Autodesk Fusion 360 part; units mm, degrees
sketch "Sketch1" plane through (0, 0, 0) normal (0, 0, 1) x (1, 0, 0)
  line L0 (-35.5, 0) -> (-21.5, 0)
  line L1 (-21.5, 0) -> (-21.5, 44)
  line L2 (-21.5, 44) -> (21.5, 44)
  line L3 (21.5, 44) -> (21.5, 0)
  line L4 (21.5, 0) -> (35.5, 0)
  line L5 (35.5, 0) -> (35.5, 4)
  line L6 (35.5, 4) -> (25.5, 4)
  line L7 (25.5, 4) -> (25.5, 47)
  line L8 (25.5, 47) -> (-25.5, 47)
  line L9 (-25.5, 47) -> (-25.5, 4)
  line L10 (-25.5, 4) -> (-35.5, 4)
  line L11 (-35.5, 4) -> (-35.5, 0)
  dimension "d1" = 43
  dimension "d2" = 21.5
  dimension "d3" = 4
  dimension "d4" = 4
  dimension "d5" = 3
  dimension "d6" = 4
  dimension "d7" = 4
  dimension "d8" = 10
  dimension "d9" = 10
  dimension "d42" = 44
  dimension "d43" = 44
extrude "Extrude1" add sketch "Sketch1" along normal blind 43
sketch "Sketch3" plane through (0, 44, 0) normal (0, -1, 0) x (1, 0, 0)
  line L0 (-21.5, 0) -> (21.5, 0)
  line L1 (21.5, 0) -> (21.5, 43)
  line L2 (21.5, 43) -> (-21.5, 43)
  line L3 (-21.5, 43) -> (-21.5, 0)
  circle A0 centre (-15.5, 6) radius 1.65
  circle A1 centre (15.5, 6) radius 1.65
  circle A2 centre (-15.5, 37) radius 1.65
  circle A3 centre (15.5, 37) radius 1.65
  dimension "d14" = 3.3
  dimension "d15" = 6
  dimension "d16" = 6
  dimension "d19" = 31
  dimension "d20" = 31
extrude "Extrude2" cut sketch "Sketch3" against normal up to surface (3 mm away) contours A0 | A1 | A2 | A3
chamfer "Chamfer1" distance 5 angle 45 2 edges at (25.5, 4, 21.5) (-25.5, 4, 21.5)
sketch "Sketch5" plane through (0, 44, 0) normal (0, -1, 0) x (1, 0, 0)
  circle A0 centre (15.5, 37) radius 1.65
  circle A1 centre (15.5, 6) radius 1.65
  circle A2 centre (-15.5, 37) radius 1.65
  circle A3 centre (-15.5, 6) radius 1.65
  line L0 (-21.5, 0) -> (21.5, 0)
  line L1 (21.5, 0) -> (21.5, 43)
  line L2 (21.5, 43) -> (-21.5, 43)
  line L3 (-21.5, 43) -> (-21.5, 0)
  circle A4 centre (0, 21) radius 13
  dimension "d25" = 26
  dimension "d26" = 21.5
extrude "Extrude3" cut sketch "Sketch5" against normal up to surface (3 mm away) contours A4
sketch "Sketch6" plane through (0, 0, 0) normal (0, -1, 0) x (1, 0, 0)
  line L0 (21.5, 0) -> (35.5, 0)
  line L1 (35.5, 0) -> (35.5, 43)
  line L2 (35.5, 43) -> (21.5, 43)
  line L3 (21.5, 43) -> (21.5, 0)
  circle A0 centre (31.5, 36.6) radius 1.65
  circle A1 centre (-31.5, 36.6) radius 1.65
  line L4 (-21.5, 0) -> (-21.5, 43)
  line L5 (-35.5, 43) -> (-21.5, 43)
  circle A2 centre (31.5, 6.6) radius 1.65
  circle A3 centre (-31.5, 6.6) radius 1.65
  dimension "d29" = 3.3
  dimension "d30" = 10
  dimension "d31" = 3.3
  dimension "d32" = 10
  dimension "d33" = 6.4
  dimension "d34" = 6.4
  dimension "d37" = 0
  dimension "d38" = -30
extrude "Extrude4" cut sketch "Sketch6" against normal blind 10 contours A0 | A1 | A2 | A3
sketch "Sketch7" plane through (0, 4, 0) normal (0, 1, 0) x (-1, 0, 0)
  arc A0 (-30.5, 7.9124) -> (-30.5, 5.2876) centre (-31.5, 6.6) ccw
  line L0 (-30.5, 7.9124) -> (-30.5, 35.2876)
  arc A1 (-30.5, 37.9124) -> (-30.5, 35.2876) centre (-31.5, 36.6) ccw
  line L1 (-30.5, 37.9124) -> (-30.5, 43)
  line L2 (-30.5, 43) -> (-35.5, 43)
  line L3 (-35.5, 43) -> (-35.5, 0)
  line L4 (-35.5, 0) -> (-30.5, 0)
  line L5 (-30.5, 0) -> (-30.5, 5.2876)
  circle A2 centre (-31.5, 6.6) radius 4
  circle A3 centre (31.5, 6.6) radius 4
  circle A4 centre (-31.5, 36.6) radius 4
  circle A5 centre (31.5, 36.6) radius 4
  dimension "d44" = 8
  dimension "d47" = 63
  dimension "d48" = 30
extrude "Extrude5" cut sketch "Sketch7" along normal blind 4 contours A0 L0 L5 A2 | A0 L0 L5 A2 | L0 A1 L1 A4 | L0 A1 L1 A4 | A3 | A5
sketch "Sketch8" plane through (25.5, 0, 0) normal (1, 0, 0) x (0, 0, -1)
  line L0 (-43, 9) -> (0, 9)
  line L1 (0, 9) -> (0, 47)
  line L2 (0, 47) -> (-43, 47)
  line L3 (-43, 47) -> (-43, 9)
  line L4 (-26.5, 37) -> (-26.5, 19)
  arc A0 (-26.5, 19) -> (-16.5, 19) centre (-21.5, 19) ccw
  line L5 (-16.5, 19) -> (-16.5, 37)
  arc A1 (-16.5, 37) -> (-26.5, 37) centre (-21.5, 37) ccw
  line L6 (-21.5, 37) -> (-21.5, 19) construction
  dimension "d51" = 18
  dimension "d52" = 10
  dimension "d53" = 21.5
extrude "Extrude6" cut sketch "Sketch8" against normal up to surface (51 mm away) contours L4 A0 L5 A1
equation "d1 = size"
equation "d2 = d1 / 2"
equation "d4 = d3"
equation "d7 = d6"
equation "d9 = d8"
equation "d10 = size"
equation "size = 43 mm"
equation "spacing = 31 mm"
equation "d15 = ( size - spacing ) / 2"
equation "d16 = d15"
equation "d26 = size / 2"
equation "d32 = d30"
equation "d34 = d33"
equation "d38 = -( size - 13 mm )"
equation "d43 = d42"
equation "d53 = ( 43 / 2 ) * 1 mm"
Check sheet for the modelled part. Datum: model origin and axes. Units: mm. A direction names the side the tool comes from. Round coordinates to 2 decimals unless told otherwise and drop trailing zeros. Order: outer loops, then holes, each group sorted by start corner. A loop starts at its lowest first (then second) coordinate and runs counter-clockwise, first axis right, second up. Notation, with made-up numbers: (-26, 2.5) -> (-16, 2.5) arc R24 cw to (-16, 34.5) -> close; hole circle Ø1 at (29.25, 67). An arc over 180 degrees is marked (long way). Use CSV: the item, a comma, the result in double quotes.
(1) Draft check along X on faces 1 (the face through (17.024, 45.479, 5.368)), 2 (the face through (28, 0, 21)), 3 (the face through (-27.5, 5.1, 6.5)), 4 (the face through (21.5, 22, 16)). Enter one of: pulls with the +X half, pulls with the -X half, needs draft (parallel to the pull), parting line crosses it, or undercut.
Worked out:
face 1,"undercut"
face 2,"needs draft"
face 3,"pulls with the -X half"
face 4,"undercut"
(2) Tool access check on faces 5 (the face through (-27.5, 5.1, 36.5)), 6 (the face through (-32.716, 1.972, 37.715)), 7 (the face through (-21.5, 22, 16)), 8 (the face through (-25.5, 28, 16)), 9 (the face through (-23, 28, 26.5)). Record the directions out of +Z, -Z, +X, -X, +Y, -Y that give a thin tool (end or side, any length) a straight path to the whole face; none if there is none.
Worked out:
face 5,"-X, +Y"
face 6,"+Y, -Y"
face 7,"+Z, -Z, -Y"
face 8,"+Z, -Z, -X, +Y"
face 9,"+X, -X"
(3) Cross-section at B-B (y = 32). Record the boundary of the cut face in (x, z).
Worked out:
outline,"(-25.5, 0) -> (-21.5, 0) -> (-21.5, 16.5) -> (-25.5, 16.5) -> close; (-25.5, 26.5) -> (-21.5, 26.5) -> (-21.5, 43) -> (-25.5, 43) -> close; (21.5, 0) -> (25.5, 0) -> (25.5, 16.5) -> (21.5, 16.5) -> close; (21.5, 26.5) -> (25.5, 26.5) -> (25.5, 43) -> (21.5, 43) -> close"
(4) Material ranges on line 1 along Z through (x, y) = (-15.5, 45.2); line 2 along Z through (x, y) = (-31.5, 2.55); line 3 along X through (y, z) = (15, 34.5), recorded low to high. Write a range as from..to.
Worked out:
line 1,"0..4.35, 7.65..35.35, 38.65..43"
line 2,"0..4.95, 8.25..34.95, 38.25..43"
line 3,"-25.5..-21.5, 21.5..25.5"
(5) Cross-section at C-C (x = -31.5). Record the boundary of the cut face in (y, z), and give its area (3 significant figures).
Worked out:
outline,"(0, 0) -> (4, 0) -> (4, 4.95) -> (0, 4.95) -> close; (0, 8.25) -> (4, 8.25) -> (4, 34.95) -> (0, 34.95) -> close; (0, 38.25) -> (4, 38.25) -> (4, 43) -> (0, 43) -> close"
area,"146 mm²"
(6) Cross-section at D-D (z = 21). Record the boundary of the cut face in (x, y).
Worked out:
outline,"(-35.5, 0) -> (-21.5, 0) -> (-21.5, 14.03) -> (-25.5, 14.03) -> (-25.5, 9) -> (-30.5, 4) -> (-35.5, 4) -> close; (-25.5, 41.97) -> (-21.5, 41.97) -> (-21.5, 44) -> (-13, 44) -> (-13, 47) -> (-25.5, 47) -> close; (13, 44) -> (21.5, 44) -> (21.5, 41.97) -> (25.5, 41.97) -> (25.5, 47) -> (13, 47) -> close; (21.5, 0) -> (35.5, 0) -> (35.5, 4) -> (30.5, 4) -> (25.5, 9) -> (25.5, 14.03) -> (21.5, 14.03) -> close"
(7) Cross-section at A-A (x = 12). Record the boundary of the cut face in (y, z), and give its area (3 significant figures).
Worked out:
outline,"(44, 0) -> (47, 0) -> (47, 16) -> (44, 16) -> close; (44, 26) -> (47, 26) -> (47, 43) -> (44, 43) -> close"
area,"99.0 mm²"
(8) Depth check by flat-ended pin: pin 1 (5.5 mm diameter, centred on x = -31.5, z = 6.6, fed in from +Y); pin 2 (19 mm diameter, centred on y = 30, z = 25.5, fed in from -X); pin 3 (12 mm diameter, centred on y = 33.5, z = 15, fed in from +X). Enter the tip coordinate at first touch or a pass-through.
Worked out:
pin 1,"y = 4"
pin 2,"x = -25.5"
pin 3,"x = 25.5"
